```python
from build123d import *

# Parameters (mm, degrees)
SKETCH1_W           = 300
SKETCH1_H           = 800
BOSS_EXTRUDE1_DEPTH = 400
SKETCH3_W           = 300
SKETCH3_H           = 180.426730866
BOSS_EXTRUDE4_DEPTH = 150
FILLET6_R           = 10
SKETCH4_R           = 30
CUT_EXTRUDE1_DEPTH  = 150
SKETCH7_W           = 251.42002043
SKETCH7_H           = 445.81306925
CUT_EXTRUDE5_DEPTH  = 170
SKETCH8_R           = 40
CUT_EXTRUDE6_DEPTH  = 80
FILLET8_R           = 10


with BuildPart() as part:
    # Sketch1 → Boss-Extrude1 (new body)
    with BuildSketch(Plane.XY):
        Rectangle(SKETCH1_W, SKETCH1_H)
    extrude(amount=BOSS_EXTRUDE1_DEPTH)

    # Sketch3 → Boss-Extrude4 (add)
    with BuildSketch(Plane(origin=(0, 400, 0), x_dir=(1, 0, 0), z_dir=(0, 1, 0))):
        with Locations((0, -90.213365433)):
            Rectangle(SKETCH3_W, SKETCH3_H)
    extrude(amount=BOSS_EXTRUDE4_DEPTH)

    # Fillet6
    fillet6_edges = [part.edges().sort_by_distance(p)[0] for p in [
        (-150, 0, 400),
        (0, -400, 400),
        (0, 400, 180.426730866),
        (-150, 475, 180.426730866),
        (150, 475, 180.426730866),
        (-150, 550, 90.213365433),
        (0, 550, 180.426730866),
        (150, 550, 90.213365433),
        (0, 550, 0),
        (150, 0, 400),
        (0, -400, 0),
        (-150, 75, 0),
        (150, 75, 0),
        (0, 400, 400),
        (150, -400, 200),
        (-150, -400, 200),
        (-150, 400, 290.213365433),
        (150, 400, 290.213365433),
    ]]
    fillet(fillet6_edges, radius=FILLET6_R)

    # Sketch4 → Cut-Extrude1 (cut)
    with BuildSketch(Plane(origin=(0, 550, 0), x_dir=(1, 0, 0), z_dir=(0, 1, 0))):
        with Locations(Location((0, -76.219748714, 0), (0, 0, 270))):
            Circle(SKETCH4_R)
    extrude(amount=-CUT_EXTRUDE1_DEPTH, mode=Mode.SUBTRACT)

    # Sketch7 → Cut-Extrude5 (cut)
    with BuildSketch(Plane(origin=(0, 0, 0), x_dir=(-1, 0, 0), z_dir=(0, 0, -1))):
        Rectangle(SKETCH7_W, SKETCH7_H)
    extrude(amount=-CUT_EXTRUDE5_DEPTH, mode=Mode.SUBTRACT)

    # Sketch8 → Cut-Extrude6 (cut)
    with BuildSketch(Plane.XZ.offset(400)):
        with Locations(Location((0, 200, 0), (0, 0, 270))):
            Circle(SKETCH8_R)
    extrude(amount=-CUT_EXTRUDE6_DEPTH, mode=Mode.SUBTRACT)

    # Fillet8
    fillet8_edges = [part.edges().sort_by_distance(p)[0] for p in [
        (-125.710010215, 0, 0),
        (0, 222.906534625, 0),
        (125.710010215, 0, 0),
        (0, -222.906534625, 0),
    ]]
    fillet(fillet8_edges, radius=FILLET8_R)


solid = part.part
```
Work out the finished part from the listing and answer in its coordinate system (mm). A direction names the side the tool comes from. Round coordinates to 2 decimals unless told otherwise and drop trailing zeros. Write each loop counter-clockwise with the first axis right and the second up, starting at its lowest first coordinate (ties: lowest second). Pieces come first, ordered by that corner, then holes.
1) A cutting plane is placed at A-A on z = 331.5. Determine the outline of the cut face in (x, y).
2) A cutting plane is placed at C-C on x = 86.5. Determine the outline of the cut face in (y, z), and give its area (3 significant figures).
3) Consider probe 1 along X at (y, z) = (-366, 200); probe 2 along Y at (x, z) = (54, 37); probe 3 along X at (y, z) = (-220, 107). Determine where each line is inside the solid, lowest interval first.
4) A cutting plane is placed at B-B on y = -119. Determine the outline of the cut face in (x, z).
5) Which of the six approach directions +Z, -Z, +X, -X, +Y, -Y give full straight-line access (tool end or side, diameter ignored) to faces 1 (the face through (-2, 400, 289)), 2 (the face through (125.71, -3, 89)), 3 (the face through (-150, 68, 203)), 4 (the face through (0, 400, 76)), 5 (the face through (1.76, -360.56, 239.96))?
6) Determine the mould class of faces 6 (the face through (-2, -400, 155)), 7 (the face through (-2, 5, 400)), 8 (the face through (2, 222.907, 89)) for opening direction Y: pulls with the +Y half, pulls with the -Y half, needs draft (parallel to the pull), parting line crosses it, or undercut.
7) A flat-ended cylindrical pin translates along its axis: P1, Ø2, axis at x = -94, z = 288, coming from the +Y side. Find the tip coordinate at first contact, or state that the pin passes through.
8) A cutting plane is placed at D-D on z = 138.5. Determine the outline of the cut face in (x, y), and give its area (3 significant figures).
Entries:
1. outline: (-150, -390) arc R10 ccw to (-140, -400) - (140, -400) arc R10 ccw to (150, -390) - (150, 390) arc R10 ccw to (140, 400) - (-140, 400) arc R10 ccw to (-150, 390) - close
2. outline: (-400, 10) arc R10 ccw to (-390, 0) - (-232.91, 0) arc R10 ccw to (-222.91, 10) - (-222.91, 170) - (222.91, 170) - (222.91, 10) arc R10 ccw to (232.91, 0) - (540, 0) arc R10 ccw to (550, 10) - (550, 170.43) arc R10 ccw to (540, 180.43) - (410, 180.43) arc R10 cw to (400, 190.43) - (400, 390) arc R10 ccw to (390, 400) - (-390, 400) arc R10 ccw to (-400, 390) - close
2. area: 271,000 mm2
3. probe 1: x = -150 to -40, 40 to 150
3. probe 2: y = -400 to -222.91, 222.91 to 550
3. probe 3: x = -150 to -125.71, 125.71 to 150
4. outline: (-150, 10) arc R10 ccw to (-140, 0) - (-135.71, 0) arc R10 ccw to (-125.71, 10) - (-125.71, 170) - (125.71, 170) - (125.71, 10) arc R10 ccw to (135.71, 0) - (140, 0) arc R10 ccw to (150, 10) - (150, 390) arc R10 ccw to (140, 400) - (-140, 400) arc R10 ccw to (-150, 390) - close
5. face 1: +Z, +X, -X, +Y
5. face 2: -Z
5. face 3: +Z, -Z, -X, +Y, -Y
5. face 4: +Y
5. face 5: -Y
6. face 6: pulls with the -Y half
6. face 7: needs draft
6. face 8: undercut
7. P1: stops at y = 400
8. outline: (-150, -390) arc R10 ccw to (-140, -400) - (140, -400) arc R10 ccw to (150, -390) - (150, 540) arc R10 ccw to (140, 550) - (-140, 550) arc R10 ccw to (-150, 540) - close; hole (-125.71, -222.91) - (125.71, -222.91) - (125.71, 222.91) - (-125.71, 222.91) - close
8. area: 173,000 mm2
